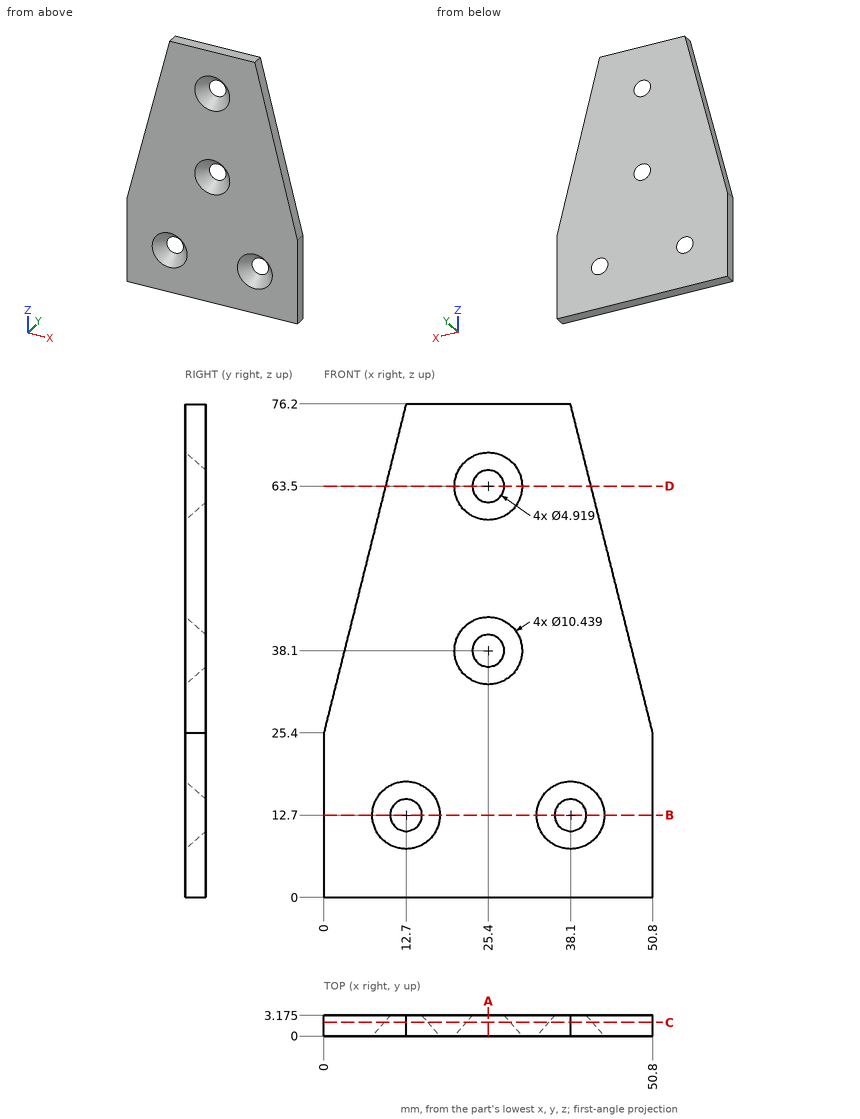
The drawing under review shows one solid part. Ordinate dimensions are in mm from its lowest x, y, z. Give positions to 0.01 mm unless a question says otherwise; leave off trailing zeros. Write each loop counter-clockwise with the first axis right and the second up, starting at its lowest first coordinate (ties: lowest second). Pieces come first, ordered by that corner, then holes. Notation, with made-up numbers: (20, 84.25) - (27, 84.25) arc R31 cw to (27, 113.25) - close; hole circle Ø7 at (-3.75, -24). An arc over 180 degrees is marked (long way). Answer in a Markdown table with one row per item. Add a question column.
1. We need section D-D on z = 63.5. Write out the cut boundary in (x, y) (1 decimal).
2. Insertion check: P1, Ø2, axis at x = 43, z = 64.5, coming from the -Y side. The pin has a flat end and moves straight along its axis. Give the tip position at first contact, or say it passes through.
3. We need section C-C on y = 2.1. Write out the cut boundary in (x, z) (1 decimal), then the cut area to 3 significant figures.
4. We need section B-B on z = 12.7. Write out the cut boundary in (x, y) (1 decimal).
5. We need section A-A on x = 25.4. Write out the cut boundary in (y, z) (1 decimal).
6. Wall thickness on line 1 along X through (y, z) = (2.3, 12) (1 decimal); line 2 along Z through (x, y) = (26, 1.05) (1 decimal); line 3 along X through (y, z) = (0.1, 38): over which ranges is each line inside the solid? List them lowest first. Write a range as [from, to].
Ans:
| question | item | result |
|---|---|---|
| 1 | outline | (9.5, 0) - (20.2, 0) - (22.9, 3.2) - (9.5, 3.2) - close; (27.9, 3.2) - (30.6, 0) - (41.3, 0) - (41.3, 3.2) - close |
| 2 | P1 | passes through |
| 3 | outline | (0, 0) - (50.8, 0) - (50.8, 25.4) - (38.1, 76.2) - (12.7, 76.2) - (0, 25.4) - close; hole circle Ø6.8 at (12.7, 12.7); hole circle Ø6.8 at (25.4, 38.1); hole circle Ø6.8 at (25.4, 63.5); hole circle Ø6.8 at (38.1, 12.7) |
| 3 | area | 3,080 mm^2 |
| 4 | outline | (0, 0) - (7.5, 0) - (10.2, 3.2) - (0, 3.2) - close; (15.2, 3.2) - (17.9, 0) - (32.9, 0) - (35.6, 3.2) - close; (40.6, 3.2) - (43.3, 0) - (50.8, 0) - (50.8, 3.2) - close |
| 5 | outline | (0, 0) - (3.2, 0) - (3.2, 35.6) - (0, 32.9) - close; (0, 43.3) - (3.2, 40.6) - (3.2, 61) - (0, 58.3) - close; (0, 68.7) - (3.2, 66) - (3.2, 76.2) - (0, 76.2) - close |
| 6 | line 1 | x = [0, 9.6], [15.8, 35], [41.2, 50.8] |
| 6 | line 2 | z = [0, 33.8], [42.4, 59.2], [67.8, 76.2] |
| 6 | line 3 | x = [3.15, 20.27], [30.53, 47.65] |
